Autodesk Inventor part; units mm, degrees
ref_plane "YZ Plane" through (0, 0, 0) normal (1, 0, 0) x (0, 1, 0)
ref_plane "XZ Plane" through (0, 0, 0) normal (0, 1, 0) x (-1, 0, 0)
ref_plane "XY Plane" through (0, 0, 0) normal (0, 0, 1) x (1, 0, 0)
sketch "Sketch28" plane through (0, 0, 0) normal (0, 0, 1) x (1, 0, 0)
  point P0 (0, 0)
sketch "Sketch29" plane through (0, 0, 0) normal (0, 0, 1) x (1, 0, 0)
  circle A0 centre (0, 0) radius 40
  dimension "d84" = 80
extrude "Extrusion25" add sketch "Sketch29" along normal blind 30
sketch "Sketch30" plane through (0, 0, 30) normal (0, 0, 1) x (1, 0, 0)
  circle A0 centre (0, 0) radius 15
  dimension "d87" = 30
extrude "Extrusion26" cut sketch "Sketch30" against normal blind 5
sketch "Sketch31" plane through (0, 0, 0) normal (0, 0, -1) x (-1, 0, 0)
  circle A0 centre (0, 0) radius 15
  dimension "d90" = 30
extrude "Extrusion27" cut sketch "Sketch31" against normal blind 5
sketch "Sketch32" plane through (0, 0, 25) normal (0, 0, 1) x (1, 0, 0)
  circle A0 centre (0, 0) radius 5
  dimension "d93" = 10
extrude "Extrusion28" cut sketch "Sketch32" against normal blind 20
sketch "Sketch33" plane through (0, 0, 25) normal (0, 0, 1) x (1, 0, 0)
  circle A0 centre (10, 0) radius 2.5
  circle A1 centre (3.0902, 9.5106) radius 2.5
  circle A2 centre (-8.0902, 5.8779) radius 2.5
  circle A3 centre (-8.0902, -5.8779) radius 2.5
  circle A4 centre (3.0902, -9.5106) radius 2.5
  point P0 (0, 0)
  dimension "d96" = 5
  dimension "d99" = 360
extrude "Extrusion29" cut sketch "Sketch33" against normal blind 20
chamfer "Chamfer1" distance 2 angle 45 2 edges at (15, 0, 0) (-15, 0, 30)
properties part number "wheel"
CAD build for the part. Positions are in the model's coordinates, mm. A direction names the side the tool comes from. Round coordinates to 2 decimals unless told otherwise and drop trailing zeros. Write each loop counter-clockwise with the first axis right and the second up, starting at its lowest first coordinate (ties: lowest second). Pieces come first, ordered by that corner, then holes. Notation, with made-up numbers: (81.5, 36) -> (118.5, 36) arc R21 cw to (118.5, 52) -> close; hole circle Ø2 at (54, 67). An arc over 180 degrees is marked (long way). Answer in a Markdown table with one row per item. Add a question column.
Item 1: Which spindle directions (+Z, -Z, +X, -X, +Y, -Y) get a long thin tool onto all of the face, cutting with end or side? Do faces 4 (the face through (14.985, 0.66, 3.479)), 5 (the face through (-14.985, 0.66, 26.521)), 6 (the face through (5.4, -10.47, 15.14)). Say none if no direction does.
Item 2: Saw through at A-A, the plane z = 16. Write the cut outline in (x, y).
Item 3: Drill centre lines: line 1 (Y direction, x = 0, z = 4); line 2 (Y direction, x = 0, z = 7); line 3 (X direction, y = -5.5, z = 4). Where is each one in solid material? Low to high. Write a range as from..to.
Item 4: Saw through at C-C, the plane y = -20.5. Write the cut outline in (x, z).
Item 5: Drop flat-ended pins along their axis: pin 1 Ø10 at (y, z) = (12, 21.5) entering from +X; pin 2 Ø10 at (y, z) = (16, 11.5) entering from -X; pin 3 Ø11.5 at (x, y) = (0, 0) entering from -Z; pin 4 Ø4.5 at (x, y) = (3.09, 9.51) entering from +Z. Give the stop position or say it passes through.
Item 6: Saw through at B-B, the plane x = -19. Write the cut outline in (y, z).
Item 7: Mould opens along X. For faces 1 (the face through (17.2, 0.6, 30)), 2 (the face through (4, 4, 5)), 3 (the face through (-8.67, 39.05, 14.79)) say: pulls with the +X half, pulls with the -X half, needs draft (parallel to the pull), parting line crosses it, or undercut.
Findings below:
| question | item | result |
|---|---|---|
| 1 | face 4 | -Z |
| 1 | face 5 | +Z |
| 1 | face 6 | +Z, -Z |
| 2 | outline | circle Ø80 at (0, 0); hole circle Ø5 at (-8.09, -5.88); hole circle Ø5 at (-8.09, 5.88); hole circle Ø10 at (0, 0); hole circle Ø5 at (3.09, -9.51); hole circle Ø5 at (3.09, 9.51); hole circle Ø5 at (10, 0) |
| 3 | line 1 | y = -40..-15, 15..40 |
| 3 | line 2 | y = -40..-5, 5..40 |
| 3 | line 3 | x = -39.62..-13.96, 13.96..39.62 |
| 4 | outline | (-34.35, 0) -> (34.35, 0) -> (34.35, 30) -> (-34.35, 30) -> close |
| 5 | pin 1 | stops at x = 39.38 |
| 5 | pin 2 | stops at x = -38.46 |
| 5 | pin 3 | stops at z = 5 |
| 5 | pin 4 | passes through |
| 6 | outline | (-35.2, 0) -> (35.2, 0) -> (35.2, 30) -> (-35.2, 30) -> close |
| 7 | face 1 | needs draft |
| 7 | face 2 | undercut |
| 7 | face 3 | parting line crosses it |
